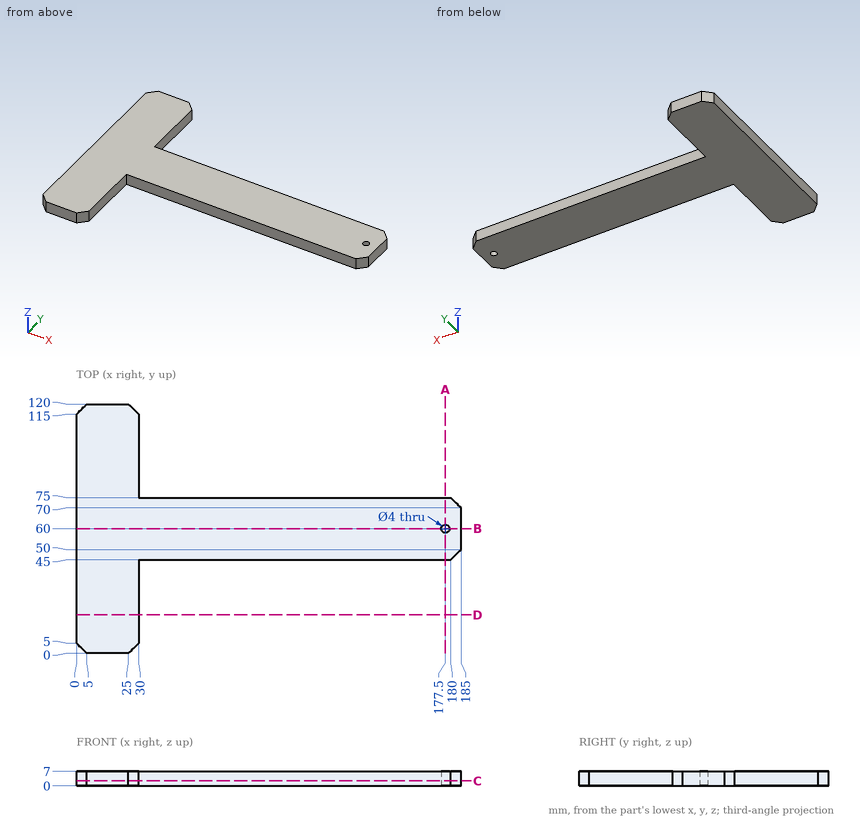
Input: dimensioned drawing with shaded views. Units: mm. Origin: part minimum x, y, z. Coordinates: 2 decimals unless noted, no trailing zeros. Loops run counter-clockwise (first coordinate to the right, second up) from the corner with the lowest first, then second, coordinate; pieces in that order, holes last. Notation, with made-up numbers: (51.5, -6) -> (72.5, -6) arc R12 cw to (72.5, 3) -> close; hole circle Ø8 at (33, 70.25). An arc over 180 degrees is marked (long way). Use a Markdown table: item, result. Add a question column.
(1) Section query A-A, the plane x = 177.5. Return loops of the section in (y, z).
(2) Pin query (flat end, axial travel): pin 1 Ø2 at (y, z) = (85.5, 3) entering from +X; pin 2 Ø3.5 at (x, z) = (135, 5) entering from +Y; pin 3 Ø3.5 at (x, z) = (84.5, 4) entering from -Y. Return the tip coordinate at first contact, or that it passes through.
(3) Section query D-D, the plane y = 18.5. Return loops of the section in (x, z).
(4) Line query: line 1 along Y through (x, z) = (177.5, 3.5); line 2 along X through (y, z) = (60, 4.5); line 3 along Y through (x, z) = (111, 4.25). Output: solid intervals per line, ascending.
(5) Section query B-B, the plane y = 60. Return loops of the section in (x, z).
(6) Section query C-C, the plane z = 2.5. Return loops of the section in (x, y).
Answer:
| question | item | result |
|---|---|---|
| 1 | outline | (45, 0) -> (58, 0) -> (58, 7) -> (45, 7) -> close; (62, 0) -> (75, 0) -> (75, 7) -> (62, 7) -> close |
| 2 | pin 1 | stops at x = 30 |
| 2 | pin 2 | stops at y = 75 |
| 2 | pin 3 | stops at y = 45 |
| 3 | outline | (0, 0) -> (30, 0) -> (30, 7) -> (0, 7) -> close |
| 4 | line 1 | y = 45 to 58, 62 to 75 |
| 4 | line 2 | x = 0 to 175.5, 179.5 to 185 |
| 4 | line 3 | y = 45 to 75 |
| 5 | outline | (0, 0) -> (175.5, 0) -> (175.5, 7) -> (0, 7) -> close; (179.5, 0) -> (185, 0) -> (185, 7) -> (179.5, 7) -> close |
| 6 | outline | (0, 5) -> (5, 0) -> (25, 0) -> (30, 5) -> (30, 45) -> (180, 45) -> (185, 50) -> (185, 70) -> (180, 75) -> (30, 75) -> (30, 115) -> (25, 120) -> (5, 120) -> (0, 115) -> close; hole circle Ø4 at (177.5, 60) |
